Part model, mm, in its own coordinate system. A direction names the side the tool comes from. Round coordinates to 2 decimals unless told otherwise and drop trailing zeros. Write each loop counter-clockwise with the first axis right and the second up, starting at its lowest first coordinate (ties: lowest second). Pieces come first, ordered by that corner, then holes.
```python
from build123d import *


with BuildPart() as part:
    # Esquisse1 → Révolution1 (revolve)
    with BuildSketch(Plane.XY, mode=Mode.PRIVATE) as r_volution1_sk:
        with BuildLine():
            ThreePointArc((22.42, 3.937322098), (20.97, 2.487322098), (22.42, 1.037322098))
            Line((22.42, 1.037322098), (22.42, 0))
            Line((22.42, 0), (23.97, 0))
            Line((23.97, 0), (3, 0))
            Line((3, 0), (3, 5))
            Line((3, 5), (3, 9))
            Line((3, 9), (8, 9))
            Line((8, 9), (8, 5))
            Line((8, 5), (23.97, 5))
            Line((23.97, 5), (22.42, 5))
            Line((22.42, 5), (22.42, 3.937322098))
        make_face()
    revolve(r_volution1_sk.sketch.rotate(Axis((0, 0, 0), (0, 1, 0)), 90), axis=Axis((0, 0, 0), (0, 1, 0)))


solid = part.part
```
Q1. Cut at C-C on y = 8.25. Write the cut outline in (x, z), plus the area to 3 significant figures.
Values follow:
outline: circle Ø16 at (0, 0); hole circle Ø6 at (0, 0)
area: 173 mm2
Q2. Which spindle directions (+Z, -Z, +X, -X, +Y, -Y) get a long thin tool onto all of the face, cutting with end or side? Do faces 1 (the cylindrical face through (7.81, 6.97, 1.73)), 2 (the flat face through (-0.1, 9, 3.4)). Say none if no direction does.
Values follow:
face 1: +Y
face 2: +Z, -Z, +X, -X, +Y
Q3. Cut at D-D on y = 3. Write the cut outline in (x, z), plus the area to 3 significant figures.
Values follow:
outline: circle Ø42.13 at (0, 0); hole circle Ø6 at (0, 0)
area: 1,370 mm2
Q4. Cut at B-B on z = 0. Write the cut outline in (x, y).
Values follow:
outline: (-22.42, 0) - (-3, 0) - (-3, 9) - (-8, 9) - (-8, 5) - (-22.42, 5) - (-22.42, 3.94) arc R1.45 cw to (-22.42, 1.04) - close; (3, 0) - (22.42, 0) - (22.42, 1.04) arc R1.45 cw to (22.42, 3.94) - (22.42, 5) - (8, 5) - (8, 9) - (3, 9) - close
Q5. Cut at A-A on x = 0. Write the cut outline in (y, z), plus the area to 3 significant figures.
Values follow:
outline: (0, -22.42) - (1.04, -22.42) arc R1.45 cw to (3.94, -22.42) - (5, -22.42) - (5, -8) - (9, -8) - (9, -3) - (0, -3) - close; (0, 3) - (9, 3) - (9, 8) - (5, 8) - (5, 22.42) - (3.94, 22.42) arc R1.45 cw to (1.04, 22.42) - (0, 22.42) - close
area: 228 mm2
Q6. Drop flat-ended pins along their axis: pin 1 (5 mm diameter, centred on x = -14.5, y = 1, fed in from -Z); pin 2 (1.5 mm diameter, centred on y = 6.5, z = 5.5, fed in from -X); pin 3 (1.5 mm diameter, centred on x = -8, y = 6, fed in from -Z). Give the stop position or say it passes through.
Values follow:
pin 1: stops at z = -18.94
pin 2: stops at x = -6.44
pin 3: stops at z = -3.38
Q7. Wall check: L1, parallel to X at y = 6, z = 0; L2, parallel to Y at x = -2, z = 18; L3, parallel to X at y = 4.5, z = 0. Give the ranges that are in metal, low to high.
Values follow:
L1: x = -8 to -3, 3 to 8
L2: y = 0 to 5
L3: x = -22.42 to -3, 3 to 22.42
